Geometry check sheet. Reference: drawing and pictorial views, mm from the part's lowest x, y, z. A direction names the side the tool comes from. Coordinates: 2 decimals unless noted, no trailing zeros. Loops run counter-clockwise (first coordinate to the right, second up) from the corner with the lowest first, then second, coordinate; pieces in that order, holes last. Notation, with made-up numbers: (36, 69.25) - (81, 69.25) arc R24 ccw to (81, 101.25) - close; hole circle Ø1 at (69, -10). An arc over 180 degrees is marked (long way). Write each question's results on one line, items separated by ' | '. Start each with the question number.
1. Gauge pin test, flat ends, axial feed: P1, Ø2.5, axis at x = 7, y = 13.05, coming from the -Z side; P2, Ø6, axis at x = 8.5, y = 9, coming from the -Z side; P3, Ø1, axis at x = 6, y = 8, coming from the +Z side; P4, Ø5, axis at x = 11.5, y = 11.5, coming from the +Z side (1 decimal). Record the tip position at first contact, or that the pin passes through.
2. Cross-section at D-D (x = 2.5). Record the cut outline in (y, z).
3. Draft check along Y on the marked faces 1, 2 and 3. Enter one of: released by +Y, released by -Y, zero draft, split by the parting line, or undercut.
4. Tool access check on the marked faces 4 and 5. Record the directions out of +Z, -Z, +X, -X, +Y, -Y that give a thin tool (end or side, any length) a straight path to the whole face; none if there is none.
5. Cross-section at C-C (x = 9.5). Record the cut outline in (y, z) (1 decimal), and give its area (3 significant figures).
6. Cross-section at A-A (x = 7). Record the cut outline in (y, z) (1 decimal).
7. Thickness scan on line 1 (Y direction, x = 7, z = 9.85); line 2 (X direction, y = 13, z = 6.25) (1 decimal); line 3 (Y direction, x = 10.75, z = 10). Record the ranges inside material, lowest first. Write a range as [from, to].
8. Cross-section at B-B (y = 4). Record the cut outline in (x, z) (1 decimal).
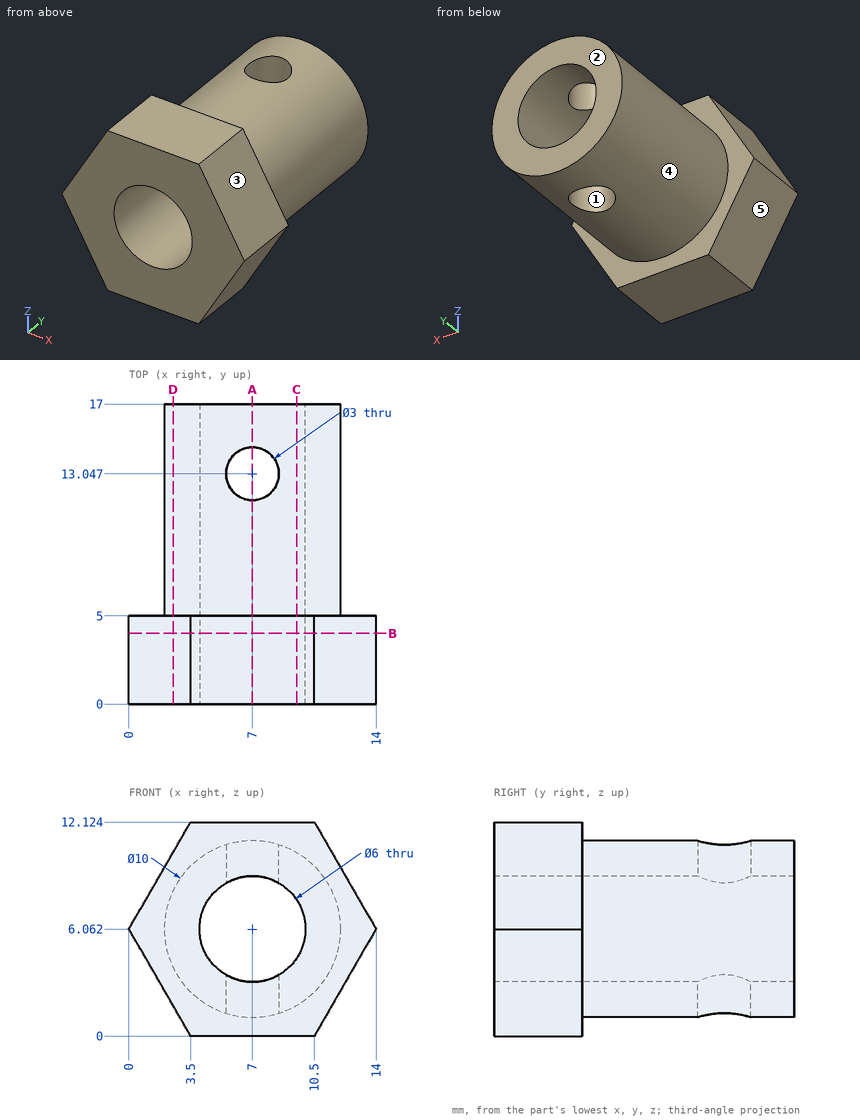
Established:
1) P1: through | P2: z = 1.06 | P3: z = 11.04 | P4: z = 10.6
2) outline: (0, 1.73) - (5, 1.73) - (5, 3.88) - (17, 3.88) - (17, 8.24) - (5, 8.24) - (5, 10.39) - (0, 10.39) - close
3) face 1: undercut | face 2: released by +Y | face 3: zero draft
4) face 4: +Y | face 5: -Z, -X, +Y, -Y
5) outline: (0, 0) - (5, 0) - (5, 1.7) - (17, 1.7) - (17, 4.4) - (0, 4.4) - close; (0, 7.7) - (17, 7.7) - (17, 10.4) - (5, 10.4) - (5, 12.1) - (0, 12.1) - close | area: 108 mm^2
6) outline: (0, 0) - (5, 0) - (5, 1.1) - (11.5, 1.1) - (11.5, 3.1) - (0, 3.1) - close; (0, 9.1) - (11.5, 9.1) - (11.5, 11.1) - (5, 11.1) - (5, 12.1) - (0, 12.1) - close; (14.5, 1.1) - (17, 1.1) - (17, 3.1) - (14.5, 3.1) - close; (14.5, 9.1) - (17, 9.1) - (17, 11.1) - (14.5, 11.1) - close
7) line 1: [0, 11.55], [14.55, 17] | line 2: [2, 4], [10, 12] | line 3: [0, 5]
8) outline: (0, 6.1) - (3.5, 0) - (10.5, 0) - (14, 6.1) - (10.5, 12.1) - (3.5, 12.1) - close; hole circle Ø6 at (7, 6.1)
